```python
from build123d import *

# Parameters (mm, degrees)
SKETCH023_R     = 1.75
PAD013_DEPTH    = 2
SKETCH024_R     = 16
PAD014_DEPTH    = 10
SKETCH025_R     = 13.25
PAD015_DEPTH    = 3
SKETCH026_R     = 12
PAD016_DEPTH    = 10
SKETCH027_R     = 5
PAD017_DEPTH    = 0.5
SKETCH028_R     = 4
PAD018_DEPTH    = 1.5
SKETCH029_R     = 2.5
PAD019_DEPTH    = 8
SKETCH030_R     = 1.25
POCKET008_DEPTH = 10
POCKET009_DEPTH = 5


with BuildPart() as part:
    # Sketch023 → Pad013 (new body)
    with BuildSketch(Plane.XY):
        with BuildLine():
            ThreePointArc((15.491933, 4), (0, 16), (-15.491933, 4))
            Line((-19, 4), (-15.491933, 4))
            ThreePointArc((-19, 4), (-23, 0), (-19, -4))
            Line((-19, -4), (-15.491933, -4))
            ThreePointArc((-15.491933, -4), (0, -16), (15.491933, -4))
            Line((15.491933, -4), (19, -4))
            ThreePointArc((19, -4), (23, 0), (19, 4))
            Line((15.491933, 4), (19, 4))
        make_face()
        with Locations((-19, 0)):
            Circle(SKETCH023_R, mode=Mode.SUBTRACT)
        with Locations((19, 0)):
            Circle(SKETCH023_R, mode=Mode.SUBTRACT)
    extrude(amount=PAD013_DEPTH)

    # Sketch024 (on Face11 of Pad013) → Pad014 (join)
    with BuildSketch(Plane(origin=(0, 0, 0), x_dir=(1, 0, 0), z_dir=(0, 0, -1))):
        Circle(SKETCH024_R)
    extrude(amount=PAD014_DEPTH)

    # Sketch025 (on Face13 of Pad014) → Pad015 (join)
    with BuildSketch(Plane(origin=(0, 0, -10), x_dir=(1, 0, 0), z_dir=(0, 0, -1))):
        Circle(SKETCH025_R)
    extrude(amount=PAD015_DEPTH)

    # Sketch026 (on Face15 of Pad015) → Pad016 (join)
    with BuildSketch(Plane(origin=(0, 0, -13), x_dir=(1, 0, 0), z_dir=(0, 0, -1))):
        Circle(SKETCH026_R)
    extrude(amount=PAD016_DEPTH)

    # Sketch027 (on Face5 of Pad016) → Pad017 (join)
    with BuildSketch(Plane.XY.offset(2)):
        with Locations((0, 8)):
            Circle(SKETCH027_R)
    extrude(amount=PAD017_DEPTH)

    # Sketch028 (on Face16 of Pad017) → Pad018 (join)
    with BuildSketch(Plane.XY.offset(2.5)):
        with Locations((0, 8)):
            Circle(SKETCH028_R)
    extrude(amount=PAD018_DEPTH)

    # Sketch029 (on Face20 of Pad018) → Pad019 (join)
    with BuildSketch(Plane.XY.offset(4)):
        with Locations((0, 8)):
            Circle(SKETCH029_R)
    extrude(amount=PAD019_DEPTH)

    # Sketch030 (on Face23 of Pad019) → Pocket008 (cut)
    with BuildSketch(Plane.XY.offset(12)):
        with Locations((0, 8)):
            Circle(SKETCH030_R)
    extrude(amount=-POCKET008_DEPTH, mode=Mode.SUBTRACT)

    # Sketch031 (on Face23 of Pocket008) → Pocket009 (cut)
    with BuildSketch(Plane.XY.offset(12)):
        with BuildLine():
            Line((2, 9.5), (2, 6.5))
            ThreePointArc((2, 6.5), (2.5, 8), (2, 9.5))
        make_face()
        with BuildLine():
            Line((-2, 9.5), (-2, 6.5))
            ThreePointArc((-2, 9.5), (-2.5, 8), (-2, 6.5))
        make_face()
    extrude(amount=-POCKET009_DEPTH, mode=Mode.SUBTRACT)


solid = part.part
```
Geometry: final body of the model. Coordinates: model frame, mm. A direction names the side the tool comes from. Round coordinates to 2 decimals unless told otherwise and drop trailing zeros. Write each loop counter-clockwise with the first axis right and the second up, starting at its lowest first coordinate (ties: lowest second). Pieces come first, ordered by that corner, then holes. Notation, with made-up numbers: M 87,73 L 92,73 A25 cw 92,101 Z; hole C 54.25,43 d10. An arc over 180 degrees is marked long. Answer in a Markdown table with one row per item. Add a question column.
(1) Cut plane C-C, the plane x = 18. Return the cut outline in (y, z), then the cut area to 3 significant figures.
(2) Cut plane B-B, the plane x = 0. Return the cut outline in (y, z), then the cut area to 4 significant figures.
(3) Draft query along Y for faces 1 (the face through (0, 0, -23)), 2 (the face through (-0.27, 6.78, 7.07)), 3 (the face through (-1.84, 9.69, 7.94)), 4 (the face through (0, 8, 2)). Return one class per face: pulls with the +Y half, pulls with the -Y half, needs draft (parallel to the pull), parting line crosses it, or undercut.
(4) Reachability of faces 5 (the face through (-6, -12, -10)), 6 (the face through (-2, 6, 4)), 7 (the face through (17, 4, 1)), 8 (the face through (-2, 8, 10)) from +Z, -Z, +X, -X, +Y, -Y: full face, straight path, thin tool, end or side. Return the list, or none.
(5) Cut plane A-A, the plane y = 0. Return the cut outline in (x, z), then the cut area to 4 significant figures.
(6) Ray query, L1, parallel to Y at x = 0, z = 7; L2, parallel to Y at x = 19, z = 0.65; L3, parallel to X at y = 0, z = -2.5. Return the intervals inside material, ascending.
(7) Contact query for flat-ended pins moving along their axis: pin 1 (6 mm diameter, centred on x = 18.5, y = 0.5, fed in from -Z); pin 2 (4 mm diameter, centred on x = -1.5, z = 5.5, fed in from +Y); pin 3 (4 mm diameter, centred on x = -0.5, y = 8, fed in from +Z); pin 4 (9.5 mm diameter, centred on x = -7, y = -4.5, fed in from +Z). Output: stop coordinate, or through.
(8) Cut plane D-D, the plane y = -5.5. Return the cut outline in (x, z), then the cut area to 3 significant figures.
Established:
| question | item | result |
|---|---|---|
| 1 | outline | M -4,0 L -1.44,0 L -1.44,2 L -4,2 Z; M 1.44,0 L 4,0 L 4,2 L 1.44,2 Z |
| 1 | area | 10.3 mm² |
| 2 | outline | M -16,-10 L -13.25,-10 L -13.25,-13 L -12,-13 L -12,-23 L 12,-23 L 12,-13 L 13.25,-13 L 13.25,-10 L 16,-10 L 16,2 L 13,2 L 13,2.5 L 12,2.5 L 12,4 L 10.5,4 L 10.5,12 L 9.25,12 L 9.25,2 L 6.75,2 L 6.75,12 L 5.5,12 L 5.5,4 L 4,4 L 4,2.5 L 3,2.5 L 3,2 L -16,2 Z |
| 2 | area | 735.5 mm² |
| 3 | face 1 | needs draft |
| 3 | face 2 | undercut |
| 3 | face 3 | parting line crosses it |
| 3 | face 4 | undercut |
| 4 | face 5 | -Z |
| 4 | face 6 | +Z |
| 4 | face 7 | +Z, -Z, +X, +Y |
| 4 | face 8 | +Z, -X, +Y, -Y |
| 5 | outline | M -23,0 L -20.75,0 L -20.75,2 L -23,2 Z; M -17.25,0 L -16,0 L -16,-10 L -13.25,-10 L -13.25,-13 L -12,-13 L -12,-23 L 12,-23 L 12,-13 L 13.25,-13 L 13.25,-10 L 16,-10 L 16,0 L 17.25,0 L 17.25,2 L -17.25,2 Z; M 20.75,0 L 23,0 L 23,2 L 20.75,2 Z |
| 5 | area | 717.5 mm² |
| 6 | L1 | 5.5 to 6.75, 9.25 to 10.5 |
| 6 | L2 | -4 to -1.75, 1.75 to 4 |
| 6 | L3 | -16 to 16 |
| 7 | pin 1 | z = -10 |
| 7 | pin 2 | y = 12 |
| 7 | pin 3 | z = 12 |
| 7 | pin 4 | z = 2 |
| 8 | outline | M -15.02,-10 L -12.05,-10 L -12.05,-13 L -10.67,-13 L -10.67,-23 L 10.67,-23 L 10.67,-13 L 12.05,-13 L 12.05,-10 L 15.02,-10 L 15.02,2 L -15.02,2 Z |
| 8 | area | 646 mm² |
